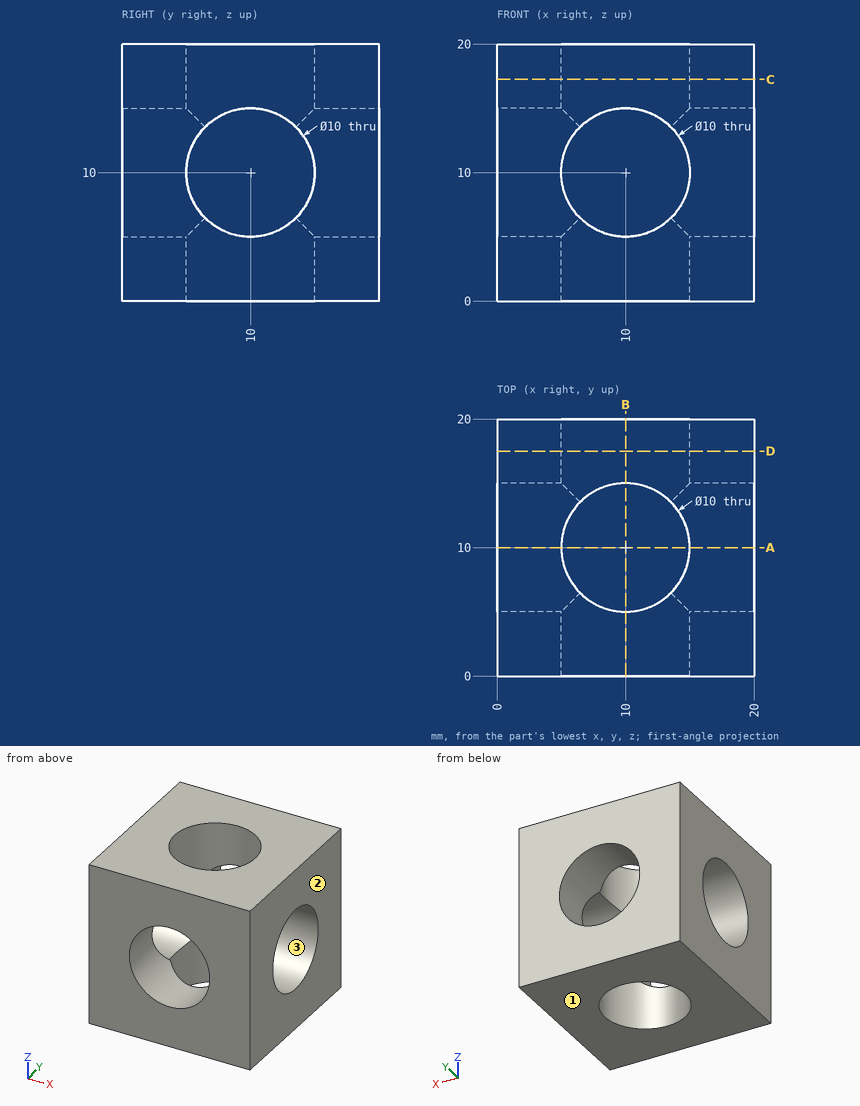
The drawing under review shows one solid part. Ordinate dimensions are in mm from its lowest x, y, z. Coordinates: 2 decimals unless noted, no trailing zeros. Write each loop counter-clockwise with the first axis right and the second up, starting at its lowest first coordinate (ties: lowest second). Pieces come first, ordered by that corner, then holes.
1) Insertion check: pin 1 (1.5 mm diameter, centred on x = 12, z = 13, fed in from +Y). The pin has a flat end and moves straight along its axis. Give the tip position at first contact, or say it passes through.
2) Mouldability with a two-part tool opening along Z and no side actions: class the marked faces 1, 2 and 3 as +Z half, -Z half, draft (parallel to the pull), parting line (faces both ways), or undercut.
3) Add section A-A (y = 10). Write out the cut boundary in (x, z), plus the area to 3 significant figures.
4) To check wall thickness, follow L1, parallel to Y at x = 10, z = 1.5. State the ranges of the line that lie inside material, in increasing order.
5) Add section C-C (z = 17.25). Write out the cut boundary in (x, y), plus the area to 3 significant figures.
Check result:
1. pin 1: passes through
2. face 1: -Z half
2. face 2: draft
2. face 3: undercut
3. outline: (0, 0) - (5, 0) - (5, 5) - (0, 5) - close; (0, 15) - (5, 15) - (5, 20) - (0, 20) - close; (15, 0) - (20, 0) - (20, 5) - (15, 5) - close; (15, 15) - (20, 15) - (20, 20) - (15, 20) - close
3. area: 100 mm2
4. L1: y = 0 to 5, 15 to 20
5. outline: (0, 0) - (20, 0) - (20, 20) - (0, 20) - close; hole circle Ø10 at (10, 10)
5. area: 321 mm2
